For this review, use the dimensioned drawing (mm, ordinates from the lowest corner) and the shaded views. A direction names the side the tool comes from. Give positions to 0.01 mm unless a question says otherwise; leave off trailing zeros. Order: outer loops, then holes, each group sorted by start corner. A loop starts at its lowest first (then second) coordinate and runs counter-clockwise, first axis right, second up. Notation, with made-up numbers: (9, 29.5) - (49, 29.5) arc R20 ccw to (49, 34.5) - close; hole circle Ø4 at (43, 23). An arc over 180 degrees is marked (long way). Use a Markdown table: item, result. Add a question column.
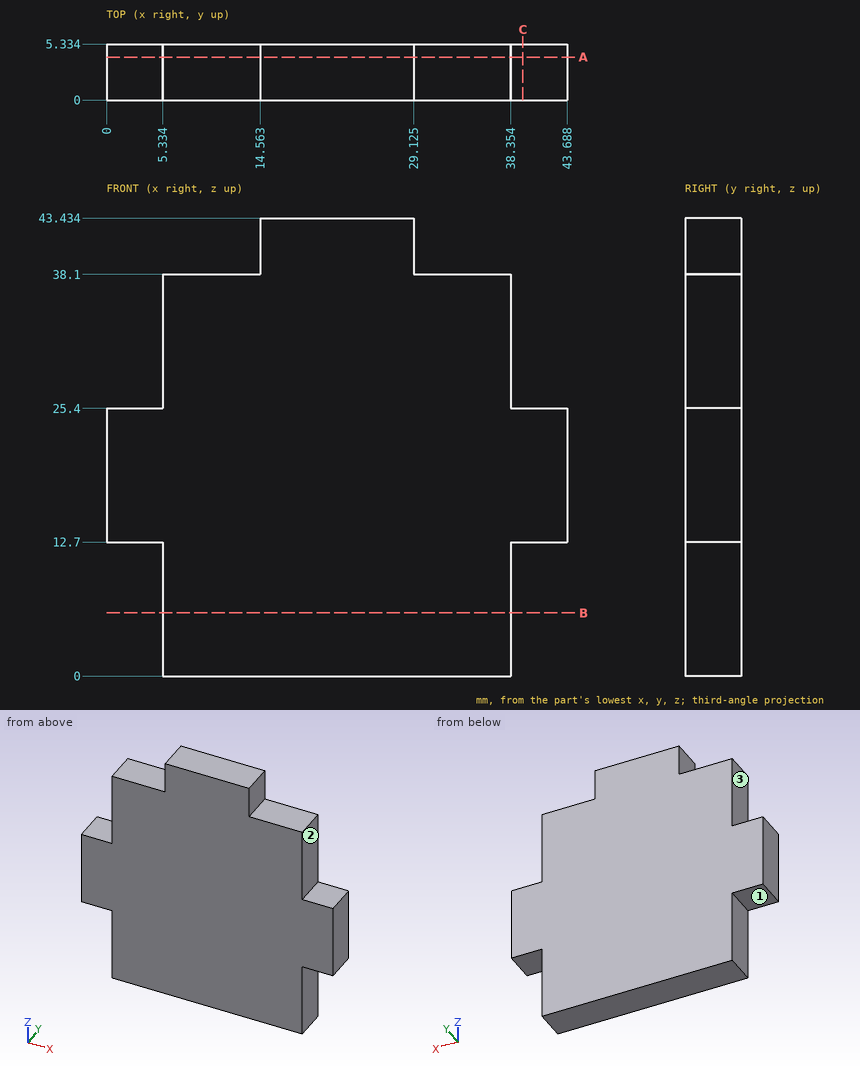
Q1. Machinability: for the marked faces 1, 2 and 3, which of the approach directions +Z, -Z, +X, -X, +Y, -Y give a long, thin tool a straight path to every point of the face, cutting with its end or side? Answer none if there is none.
Q2. Wall thickness on probe 1 along Z at (x, y) = (2.5, 1.4); probe 2 along X at (y, z) = (2.65, 9); probe 3 along Z at (x, y) = (12, 4.2): over which ranges is each line inside the solid? List them lowest first.
Q3. We need section A-A (y = 4.1). Write out the cut boundary in (x, z) (1 decimal).
Q4. We need section B-B (z = 6). Write out the cut boundary in (x, y), plus the area to 3 significant figures.
Q5. We need section C-C (x = 39.5). Write out the cut boundary in (y, z).
Q6. Clearance check with flat-ended pins moving along their axes: P1, Ø1.6, axis at y = 2.5, z = 42, coming from the +X side (1 decimal); P2, Ø2.5, axis at y = 2, z = 29.5, coming from the -X side; P3, Ø2.5, axis at x = 41.5, y = 3.5, coming from the -Z side. State where each tip first meets the part, or that it passes through.
Here are the results:
| question | item | result |
|---|---|---|
| 1 | face 1 | -Z, -X, +Y, -Y |
| 1 | face 2 | +Z, +X, +Y, -Y |
| 1 | face 3 | +Z, -X, +Y, -Y |
| 2 | probe 1 | 12.7 to 25.4 |
| 2 | probe 2 | 5.33 to 38.35 |
| 2 | probe 3 | 0 to 38.1 |
| 3 | outline | (0, 12.7) - (5.3, 12.7) - (5.3, 0) - (38.4, 0) - (38.4, 12.7) - (43.7, 12.7) - (43.7, 25.4) - (38.4, 25.4) - (38.4, 38.1) - (29.1, 38.1) - (29.1, 43.4) - (14.6, 43.4) - (14.6, 38.1) - (5.3, 38.1) - (5.3, 25.4) - (0, 25.4) - close |
| 4 | outline | (5.33, 0) - (38.35, 0) - (38.35, 5.33) - (5.33, 5.33) - close |
| 4 | area | 176 mm2 |
| 5 | outline | (0, 12.7) - (5.33, 12.7) - (5.33, 25.4) - (0, 25.4) - close |
| 6 | P1 | x = 29.1 |
| 6 | P2 | x = 5.33 |
| 6 | P3 | z = 12.7 |
